Input: part model. Units: mm. Frame: model coordinates. Coordinates: 2 decimals unless noted, no trailing zeros. Order: outer loops, then holes, each group sorted by start corner. A loop starts at its lowest first (then second) coordinate and runs counter-clockwise, first axis right, second up. Notation, with made-up numbers: (37, -33) -> (48, -33) arc R10 cw to (48, -15) -> close; hole circle Ø2 at (4.25, 33.25). An arc over 180 degrees is marked (long way). Use one line per item in the form item = value. Start each with the question number.
1) Ray query, line 1 along Z through (x, y) = (-355, 22); line 2 along X through (y, z) = (50, 9669); line 3 along Z through (x, y) = (-352, 64). Return the intervals inside material, ascending.
2) Section query B-B on x = -355. Output: boundary loops of the cut face in (y, z).
3) Section query A-A on z = 9669. Output: boundary loops of the cut face in (x, y).
4) Pin query (flat end, axial travel): pin 1 (8.5 mm diameter, centred on x = -355, z = 9669, fed in from +Y). Return the tip coordinate at first contact, or that it passes through.
Autodesk Inventor part; units mm, degrees
ref_plane "YZ Plane" through (0, 0, 0) normal (1, 0, 0) x (0, 1, 0)
ref_plane "XZ Plane" through (0, 0, 0) normal (0, 1, 0) x (-1, 0, 0)
ref_plane "XY Plane" through (0, 0, 0) normal (0, 0, 1) x (1, 0, 0)
sketch "Boceto1" plane through (0, 0, 0) normal (0, 1, 0) x (-1, 0, 0)
  line L0 (280, 9744) -> (430, 9744)
  line L1 (430, 9744) -> (430, 9594)
  line L2 (430, 9594) -> (280, 9594)
  line L3 (280, 9594) -> (280, 9744)
  point P0 (0, 0)
  dimension "d1" = 150
  dimension "d2" = 150
  dimension "d3" = 150
extrude "Extrusión1" add sketch "Boceto1" along normal blind 75
sketch "Boceto2" plane through (0, 75, 0) normal (0, 1, 0) x (1, 0, 0)
  point P0 (0, 0)
sketch "Boceto3" plane through (0, 75, 0) normal (0, 1, 0) x (1, 0, 0)
  point P0 (0, 0)
sketch "Boceto4" plane through (0, 75, 0) normal (0, 1, 0) x (1, 0, 0)
  circle A0 centre (-355, -9669) radius 7.25
  point P0 (0, 0)
  point P1 (-430, -9744)
  dimension "d8" = 14.5
hole "Agujero1" at (-355, 75, 9669) direction (0, -1, 0) diameter 14.5 end through all
fillet "Empalme1" radius 2 12 edges at (-280, 75, 9669) (-280, 37.5, 9594) (-355, 75, 9594) (-430, 37.5, 9594) (-430, 75, 9669) (-355, 75, 9744) (-430, 37.5, 9744) (-280, 37.5, 9744) (-280, 0, 9669) (-355, 0, 9594) (-430, 0, 9669) (-355, 0, 9744)
properties part number "robotico"
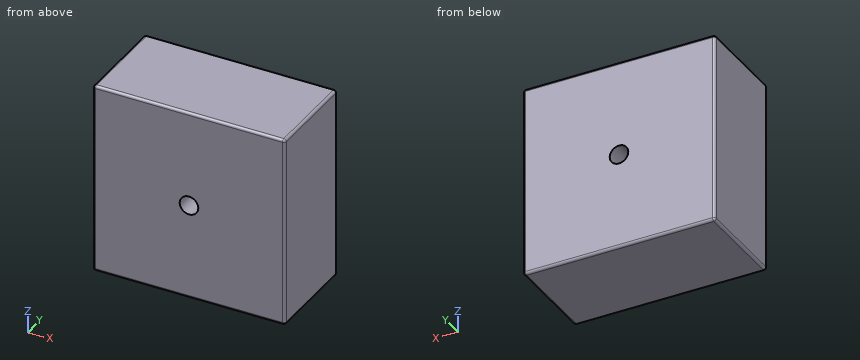
Answers below:
q1.line_1 = 9594 to 9661.75, 9676.25 to 9744
q1.line_2 = -430 to -362.25, -347.75 to -280
q1.line_3 = 9594 to 9662.4, 9675.6 to 9744
q2.outline = (0, 9596) arc R2 ccw to (2, 9594) -> (73, 9594) arc R2 ccw to (75, 9596) -> (75, 9661.75) -> (0, 9661.75) -> close; (0, 9676.25) -> (75, 9676.25) -> (75, 9742) arc R2 ccw to (73, 9744) -> (2, 9744) arc R2 ccw to (0, 9742) -> close
q3.outline = (-430, 2) arc R2 ccw to (-428, 0) -> (-362.25, 0) -> (-362.25, 75) -> (-428, 75) arc R2 ccw to (-430, 73) -> close; (-347.75, 0) -> (-282, 0) arc R2 ccw to (-280, 2) -> (-280, 73) arc R2 ccw to (-282, 75) -> (-347.75, 75) -> close
q4.pin_1 = through
